Input: part model. Units: mm. Frame: model coordinates. Face numbers are marked on the shaded views. A direction names the side the tool comes from. Coordinates: 2 decimals unless noted, no trailing zeros. Order: outer loops, then holes, each group sorted by start corner. A loop starts at its lowest first (then second) coordinate and runs counter-clockwise, first axis right, second up. Notation, with made-up numbers: (-24.5, 38.25) -> (-8.5, 38.25) arc R11 ccw to (-8.5, 43.25) -> close; hole circle Ø1 at (47.25, -23.5). An arc over 180 degrees is marked (long way). One line per question, with ' | ' between items.
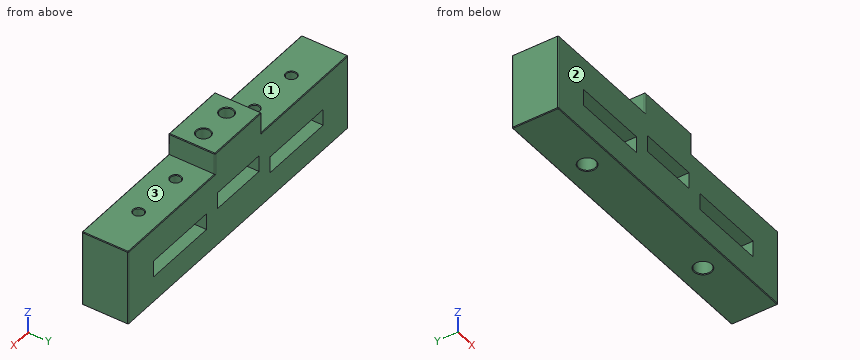
```python
from build123d import *

# Parameters (mm, degrees)
SKETCH_W        = 18
SKETCH_H        = 5
SKETCH_W_2      = 23
PAD_DEPTH       = 14
SKETCH001_R     = 2
POCKET_DEPTH    = 17.5
SKETCH002_R     = 1.5
POCKET001_DEPTH = 14
SKETCH005_R     = 1.5
POCKET002_DEPTH = 14
SKETCH006_R     = 2.5
POCKET003_DEPTH = 20
FILLET_R        = 0.3
CHAMFER_SIZE    = 0.2
CHAMFER001_SIZE = 0.2
CHAMFER002_SIZE = 0.2
CHAMFER003_SIZE = 0.2
CHAMFER004_SIZE = 0.2


with BuildPart() as part:
    # Sketch → Pad (new body)
    with BuildSketch(Plane.XZ):
        Polygon((-47.5, 0), (47.5, 0), (47.5, 23), (10, 23), (10, 29.5), (-10, 29.5), (-10, 23), (-47.5, 23), align=None)
        with Locations((0, 14)):
            Rectangle(SKETCH_W, SKETCH_H, mode=Mode.SUBTRACT)
        with Locations((-25.2, 10.5)):
            Rectangle(SKETCH_W_2, SKETCH_H, mode=Mode.SUBTRACT)
        with Locations((25.2, 10.5)):
            Rectangle(SKETCH_W_2, SKETCH_H, mode=Mode.SUBTRACT)
    extrude(amount=PAD_DEPTH)

    # Sketch001 → Pocket (cut)
    with BuildSketch(Plane(origin=(0, 0, 29.5), x_dir=(-1, 0, 0), z_dir=(0, 0, 1))):
        with Locations((-5, 7)):
            Circle(SKETCH001_R)
        with Locations((5, 7)):
            Circle(SKETCH001_R)
    extrude(amount=-POCKET_DEPTH, mode=Mode.SUBTRACT)

    # Sketch002 → Pocket001 (cut)
    with BuildSketch(Plane(origin=(0, 0, 23), x_dir=(-1, 0, 0), z_dir=(0, 0, 1))):
        with Locations((-17, 7)):
            Circle(SKETCH002_R)
        with Locations((-33, 7)):
            Circle(SKETCH002_R)
    extrude(amount=-POCKET001_DEPTH, mode=Mode.SUBTRACT)

    # Sketch005 → Pocket002 (cut)
    with BuildSketch(Plane(origin=(0, 0, 23), x_dir=(-1, 0, 0), z_dir=(0, 0, 1))):
        with Locations((33, 7)):
            Circle(SKETCH005_R)
        with Locations((17, 7)):
            Circle(SKETCH005_R)
    extrude(amount=-POCKET002_DEPTH, mode=Mode.SUBTRACT)

    # Sketch006 → Pocket003 (cut)
    with BuildSketch(Plane(origin=(0, 0, 0), x_dir=(1, 0, 0), z_dir=(0, 0, -1))):
        with Locations((-25, 7)):
            Circle(SKETCH006_R)
        with Locations((25, 7)):
            Circle(SKETCH006_R)
    extrude(amount=-POCKET003_DEPTH, mode=Mode.SUBTRACT)

    # Fillet
    fillet_edges = [part.edges().sort_by_distance(p)[0] for p in [
        (-47.5, -14, 11.5),
        (-47.5, 0, 11.5),
        (47.5, 0, 11.5),
        (47.5, -14, 11.5),
        (10, -14, 26.25),
        (10, 0, 26.25),
        (-10, 0, 26.25),
        (-10, -14, 26.25),
    ]]
    fillet(fillet_edges, radius=FILLET_R)

    # Chamfer
    chamfer_edges = [part.edges().sort_by_distance(p)[0] for p in [
        (-9.912132, -13.912132, 29.5),
        (-10, -7, 29.5),
        (-9.912132, -0.087868, 29.5),
        (0, 0, 29.5),
        (9.912132, -0.087868, 29.5),
        (10, -7, 29.5),
        (9.912132, -13.912132, 29.5),
        (0, -14, 29.5),
    ]]
    chamfer(chamfer_edges, length=CHAMFER_SIZE)

    # Chamfer001
    chamfer001_edges = [part.edges().sort_by_distance(p)[0] for p in [
        (28.6, -14, 23),
        (47.5, -7, 23),
        (47.412132, -13.912132, 23),
        (47.412132, -0.087868, 23),
        (28.6, 0, 23),
        (9.85, -14, 23),
        (9.85, 0, 23),
    ]]
    chamfer(chamfer001_edges, length=CHAMFER001_SIZE)

    # Chamfer002
    chamfer002_edges = [part.edges().sort_by_distance(p)[0] for p in [
        (-9.85, -14, 23),
        (-28.6, -14, 23),
        (-47.412132, -13.912132, 23),
        (-47.5, -7, 23),
        (-9.85, 0, 23),
        (-28.6, 0, 23),
        (-47.412132, -0.087868, 23),
    ]]
    chamfer(chamfer002_edges, length=CHAMFER002_SIZE)

    # Chamfer003
    chamfer003_edges = [part.edges().sort_by_distance(p)[0] for p in [
        (-47.412132, -13.912132, 0),
        (0, -14, 0),
        (-47.5, -7, 0),
        (-47.412132, -0.087868, 0),
        (0, 0, 0),
        (47.412132, -0.087868, 0),
        (47.5, -7, 0),
        (47.412132, -13.912132, 0),
        (22.5, -7, 0),
        (-27.5, -7, 0),
    ]]
    chamfer(chamfer003_edges, length=CHAMFER003_SIZE)

    # Chamfer004
    chamfer004_edges = [part.edges().sort_by_distance(p)[0] for p in [
        (34.5, -7, 23),
        (18.5, -7, 23),
        (7, -7, 29.5),
        (-3, -7, 29.5),
        (-15.5, -7, 23),
        (-31.5, -7, 23),
    ]]
    chamfer(chamfer004_edges, length=CHAMFER004_SIZE)


solid = part.part
```
1. Cut plane B-B, the plane x = -25. Return loops of the section in (y, z).
Recorded:
outline: (-14, 0.2) -> (-13.8, 0) -> (-9.7, 0) -> (-9.5, 0.2) -> (-9.5, 8) -> (-14, 8) -> close; (-14, 13) -> (-9.5, 13) -> (-9.5, 20) -> (-4.5, 20) -> (-4.5, 13) -> (0, 13) -> (0, 22.8) -> (-0.2, 23) -> (-13.8, 23) -> (-14, 22.8) -> close; (-4.5, 0.2) -> (-4.3, 0) -> (-0.2, 0) -> (0, 0.2) -> (0, 8) -> (-4.5, 8) -> close
2. Cut plane D-D, the plane y = -10.75. Return loops of the section in (x, z).
Recorded:
outline: (-47.5, 0.2) -> (-47.3, 0) -> (47.3, 0) -> (47.5, 0.2) -> (47.5, 22.8) -> (47.3, 23) -> (10, 23) -> (10, 29.3) -> (9.8, 29.5) -> (-9.8, 29.5) -> (-10, 29.3) -> (-10, 23) -> (-47.3, 23) -> (-47.5, 22.8) -> close; hole (-36.7, 8) -> (-13.7, 8) -> (-13.7, 13) -> (-36.7, 13) -> close; hole (-9, 11.5) -> (9, 11.5) -> (9, 16.5) -> (-9, 16.5) -> close; hole (13.7, 8) -> (36.7, 8) -> (36.7, 13) -> (13.7, 13) -> close
3. Access query for the marked faces 1, 2 and 3. Directions: +Z, -Z, +X, -X, +Y, -Y. A direction counts if a zero-diameter tool reaches every point of the face in a straight line with its end or side. Return the directions, or none.
Recorded:
face 1: +Z, -X, +Y, -Y | face 2: +Z, -Z, +X, -X, -Y | face 3: +Z, +X, +Y, -Y
4. Pin query (flat end, axial travel): pin 1 Ø3 at (x, y) = (-25, -7) entering from -Z; pin 2 Ø4 at (x, y) = (24, -9.5) entering from +Z; pin 3 Ø1.9 at (y, z) = (-5.5, 26.5) entering from -X. Return the tip coordinate at first contact, or that it passes through.
Recorded:
pin 1: stops at z = 20 | pin 2: stops at z = 23 | pin 3: stops at x = -10
5. Ray query, line 1 (X direction, y = -7, z = 26.75); line 2 (Z direction, x = -14.5, y = -6.25); line 3 (Y direction, x = -17, z = 19.5). Return the intervals inside material, ascending. Write a range as [from, to].
Recorded:
line 1: x = [-10, -7], [-3, 3], [7, 10] | line 2: z = [0, 8], [13, 23] | line 3: y = [-14, -8.5], [-5.5, 0]
6. Cut plane A-A, the plane z = 15.5. Return loops of the section in (x, y), and give its area (3 significant figures).
Recorded:
outline: (-47.5, -13.7) arc R0.3 ccw to (-47.2, -14) -> (-9, -14) -> (-9, 0) -> (-47.2, 0) arc R0.3 ccw to (-47.5, -0.3) -> close; (9, -14) -> (47.2, -14) arc R0.3 ccw to (47.5, -13.7) -> (47.5, -0.3) arc R0.3 ccw to (47.2, 0) -> (9, 0) -> close; hole circle Ø3 at (-33, -7); hole circle Ø5 at (-25, -7); hole circle Ø3 at (-17, -7); hole circle Ø3 at (17, -7); hole circle Ø5 at (25, -7); hole circle Ø3 at (33, -7) | area: 1,010 mm^2
7. Cut plane C-C, the plane x = 0. Return loops of the section in (y, z), and give its area (3 significant figures).
Recorded:
outline: (-14, 0.2) -> (-13.8, 0) -> (-0.2, 0) -> (0, 0.2) -> (0, 11.5) -> (-14, 11.5) -> close; (-14, 16.5) -> (0, 16.5) -> (0, 29.3) -> (-0.2, 29.5) -> (-13.8, 29.5) -> (-14, 29.3) -> close | area: 343 mm^2
